Job drawing, mm, ordinate dimensions from the low corner. One solid piece. Coordinates: 2 decimals unless noted, no trailing zeros. Write each loop counter-clockwise with the first axis right and the second up, starting at its lowest first coordinate (ties: lowest second). Pieces come first, ordered by that corner, then holes. Notation, with made-up numbers: (86.25, -9.5) - (116.25, -9.5) arc R25 ccw to (116.25, 13.5) - close; hole circle Ø9 at (-19.75, -8). An arc over 180 degrees is marked (long way). Use a Markdown table: item, result.
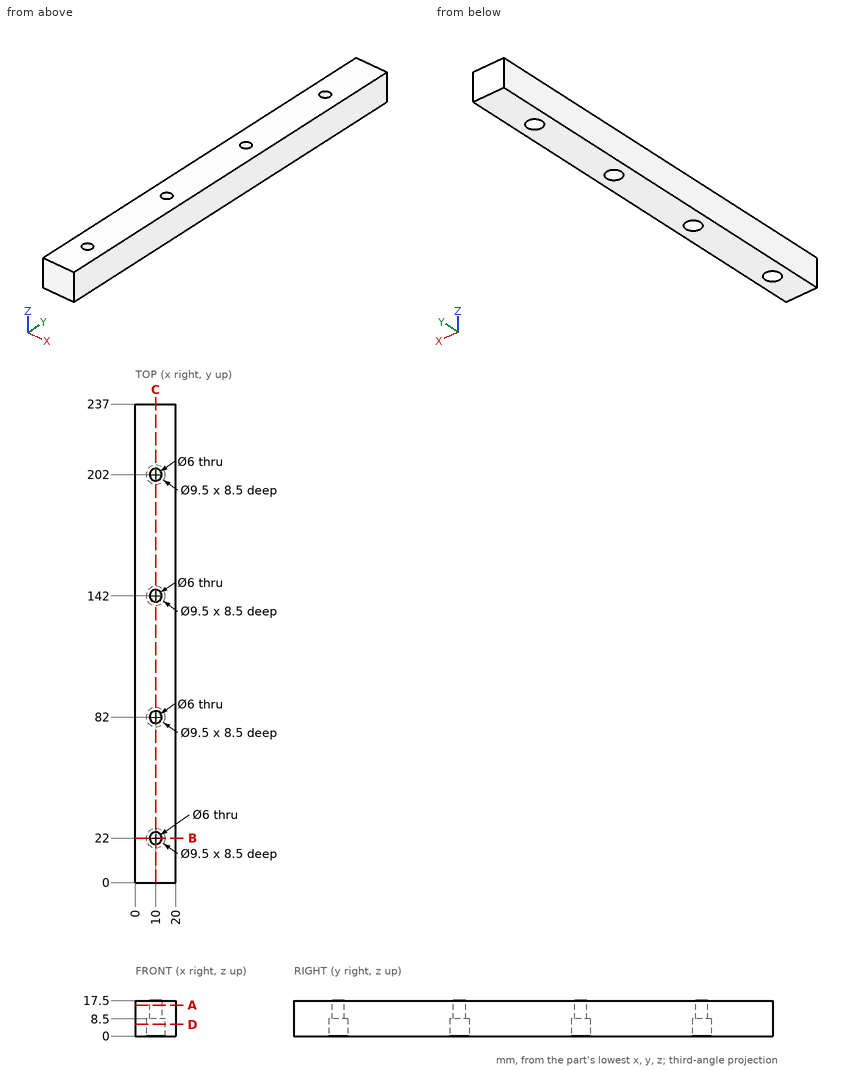
Item 1: Drop flat-ended pins along their axis: P1, Ø8, axis at x = 10, y = 22, coming from the -Z side; P2, Ø3.5, axis at x = 10, y = 142, coming from the +Z side. Give the stop position or say it passes through.
From the geometry:
| item | result |
|---|---|
| P1 | z = 8.5 |
| P2 | through |
Item 2: Band-saw the part on C-C, the plane x = 10. Count the separate pieces of the cut face and the enclosed holes in it, then the cut area to 3 significant figures.
From the geometry:
| item | result |
|---|---|
| separate pieces | 5 |
| enclosed holes | 0 |
| area | 3,610 mm^2 |
Item 3: Drill centre lines: probe 1 along Y at (x, z) = (10, 5.25); probe 2 along Y at (x, z) = (10, 14.5); probe 3 along X at (y, z) = (142, 13.5). Where is each one in solid material? Low to high.
From the geometry:
| item | result |
|---|---|
| probe 1 | 0 to 17.25, 26.75 to 77.25, 86.75 to 137.25, 146.75 to 197.25, 206.75 to 237 |
| probe 2 | 0 to 19, 25 to 79, 85 to 139, 145 to 199, 205 to 237 |
| probe 3 | 0 to 7, 13 to 20 |
Item 4: Band-saw the part on B-B, the plane y = 22. Give the cut face in (x, z), then the cut area to 3 significant figures.
From the geometry:
| item | result |
|---|---|
| outline | (0, 0) - (5.25, 0) - (5.25, 8.5) - (7, 8.5) - (7, 17.5) - (0, 17.5) - close; (13, 8.5) - (14.75, 8.5) - (14.75, 0) - (20, 0) - (20, 17.5) - (13, 17.5) - close |
| area | 215 mm^2 |
Item 5: Band-saw the part on D-D, the plane z = 5.75. Give the cut face in (x, y), then the cut area to 3 significant figures.
From the geometry:
| item | result |
|---|---|
| outline | (0, 0) - (20, 0) - (20, 237) - (0, 237) - close; hole circle Ø9.5 at (10, 22); hole circle Ø9.5 at (10, 82); hole circle Ø9.5 at (10, 142); hole circle Ø9.5 at (10, 202) |
| area | 4,460 mm^2 |
Item 6: Band-saw the part on A-A, the plane z = 15.25. Give the cut face in (x, y), then the cut area to 3 significant figures.
From the geometry:
| item | result |
|---|---|
| outline | (0, 0) - (20, 0) - (20, 237) - (0, 237) - close; hole circle Ø6 at (10, 22); hole circle Ø6 at (10, 82); hole circle Ø6 at (10, 142); hole circle Ø6 at (10, 202) |
| area | 4,630 mm^2 |
